from build123d import *

# Parameters (mm, degrees)
BASE_W                       = 90
BASE_H                       = 61
BASE_BLOCK_DEPTH             = 2.05
OUTER_PIN_STAND_DEPTH        = 1.4
OUTER_PIN_STAND_DEPTH_BACK   = 0.5
OUTER_PIN_R                  = 3
OUTER_PIN_STAND_2_DEPTH      = 1.4
OUTER_PIN_STAND_2_DEPTH_BACK = 0.5
OUTER_PIN_STAND_3_DEPTH      = 1.4
OUTER_PIN_STAND_3_DEPTH_BACK = 0.5
OUTER_PIN_STAND_4_DEPTH      = 1.4
OUTER_PIN_STAND_4_DEPTH_BACK = 0.5
INNER_PIN_STAND_DEPTH        = 2.6
INNER_PIN_STAND_DEPTH_BACK   = 0.5
SKETCH3_R                    = 1.25
INNER_PIN_STAND_2_DEPTH      = 2.6
INNER_PIN_STAND_2_DEPTH_BACK = 0.5
INNER_PIN_STAND_3_DEPTH      = 2.6
INNER_PIN_STAND_3_DEPTH_BACK = 0.5
INNER_PIN_STAND_4_DEPTH      = 2.6
INNER_PIN_STAND_4_DEPTH_BACK = 0.5
HOLES_DEPTH                  = 5
HOLES_DEPTH_BACK             = 5
SKETCH5_R                    = 1.75
HOLES_2_DEPTH                = 5
HOLES_2_DEPTH_BACK           = 5
SKETCH5_R_2                  = 1.775


with BuildPart() as part:
    # Base → Base Block (new body)
    with BuildSketch(Plane.XY):
        Rectangle(BASE_W, BASE_H)
    extrude(amount=-BASE_BLOCK_DEPTH)


with BuildPart() as body_2:
    # Outer Pin → Outer Pin Stand (new, two sides: drawn at the far end of the back side and taken through both)
    with BuildSketch(Plane.XY.offset(-OUTER_PIN_STAND_DEPTH_BACK)):
        with Locations((-39, 24.5)):
            Circle(OUTER_PIN_R)
    extrude(amount=OUTER_PIN_STAND_DEPTH + OUTER_PIN_STAND_DEPTH_BACK)


with BuildPart() as body_3:
    # Outer Pin → Outer Pin Stand 2 (new, two sides: drawn at the far end of the back side and taken through both)
    with BuildSketch(Plane.XY.offset(-OUTER_PIN_STAND_2_DEPTH_BACK)):
        with Locations((-39, -24.5)):
            Circle(OUTER_PIN_R)
    extrude(amount=OUTER_PIN_STAND_2_DEPTH + OUTER_PIN_STAND_2_DEPTH_BACK)


with BuildPart() as body_4:
    # Outer Pin → Outer Pin Stand 3 (new, two sides: drawn at the far end of the back side and taken through both)
    with BuildSketch(Plane.XY.offset(-OUTER_PIN_STAND_3_DEPTH_BACK)):
        with Locations((19.1, -24.5)):
            Circle(OUTER_PIN_R)
    extrude(amount=OUTER_PIN_STAND_3_DEPTH + OUTER_PIN_STAND_3_DEPTH_BACK)


with BuildPart() as body_5:
    # Outer Pin → Outer Pin Stand 4 (new, two sides: drawn at the far end of the back side and taken through both)
    with BuildSketch(Plane.XY.offset(-OUTER_PIN_STAND_4_DEPTH_BACK)):
        with Locations((19.1, 24.5)):
            Circle(OUTER_PIN_R)
    extrude(amount=OUTER_PIN_STAND_4_DEPTH + OUTER_PIN_STAND_4_DEPTH_BACK)


with BuildPart() as body_6:
    # Sketch3 → Inner Pin Stand (new, two sides: drawn at the far end of the back side and taken through both)
    with BuildSketch(Plane.XY.offset(-INNER_PIN_STAND_DEPTH_BACK)):
        with Locations((-39, 24.5)):
            Circle(SKETCH3_R)
    extrude(amount=INNER_PIN_STAND_DEPTH + INNER_PIN_STAND_DEPTH_BACK)


with BuildPart() as body_7:
    # Sketch3 → Inner Pin Stand 2 (new, two sides: drawn at the far end of the back side and taken through both)
    with BuildSketch(Plane.XY.offset(-INNER_PIN_STAND_2_DEPTH_BACK)):
        with Locations((19.1, 24.5)):
            Circle(SKETCH3_R)
    extrude(amount=INNER_PIN_STAND_2_DEPTH + INNER_PIN_STAND_2_DEPTH_BACK)


with BuildPart() as body_8:
    # Sketch3 → Inner Pin Stand 3 (new, two sides: drawn at the far end of the back side and taken through both)
    with BuildSketch(Plane.XY.offset(-INNER_PIN_STAND_3_DEPTH_BACK)):
        with Locations((19.1, -24.5)):
            Circle(SKETCH3_R)
    extrude(amount=INNER_PIN_STAND_3_DEPTH + INNER_PIN_STAND_3_DEPTH_BACK)


with BuildPart() as body_9:
    # Sketch3 → Inner Pin Stand 4 (new, two sides: drawn at the far end of the back side and taken through both)
    with BuildSketch(Plane.XY.offset(-INNER_PIN_STAND_4_DEPTH_BACK)):
        with Locations((-39, -24.5)):
            Circle(SKETCH3_R)
    extrude(amount=INNER_PIN_STAND_4_DEPTH + INNER_PIN_STAND_4_DEPTH_BACK)


with BuildPart() as body_10:
    # Sketch5 → Holes (new, two sides: drawn at the far end of the back side and taken through both)
    with BuildSketch(Plane.XY.offset(-HOLES_DEPTH_BACK)):
        with Locations((-39, -18.72)):
            Circle(SKETCH5_R)
    extrude(amount=HOLES_DEPTH + HOLES_DEPTH_BACK)


with BuildPart() as body_11:
    # Sketch5 → Holes 2 (new, two sides: drawn at the far end of the back side and taken through both)
    with BuildSketch(Plane.XY.offset(-HOLES_2_DEPTH_BACK)):
        with Locations((19.1, 18.86871886)):
            Circle(SKETCH5_R_2)
    extrude(amount=HOLES_2_DEPTH + HOLES_2_DEPTH_BACK)


with BuildPart() as part_1:
    add(part.part)

    # Combine1: union body 2, body 6, body 5, body 7, body 4, body 8, body 3, body 9
    add(body_2.part)
    add(body_6.part)
    add(body_5.part)
    add(body_7.part)
    add(body_4.part)
    add(body_8.part)
    add(body_3.part)
    add(body_9.part)

    # Combine2: cut body 11, body 10
    add(body_11.part, mode=Mode.SUBTRACT)
    add(body_10.part, mode=Mode.SUBTRACT)


solid = part_1.part
Geometry check sheet. Reference: the model listing, model coordinates, mm. A direction names the side the tool comes from. Round coordinates to 2 decimals unless told otherwise and drop trailing zeros. Order: outer loops, then holes, each group sorted by start corner. A loop starts at its lowest first (then second) coordinate and runs counter-clockwise, first axis right, second up. Notation, with made-up numbers: (-16.75, -39.75) - (19.25, -39.75) arc R23 ccw to (19.25, -31.75) - close; hole circle Ø3 at (-14, 19.25). An arc over 180 degrees is marked (long way). One line per question, with ' | ' between items. Start each with the question number.
(1) Sectioned sample at A-A on y = -18.72. Record the cut outline in (x, z).
(2) Sectioned sample at D-D on x = 5. Record the cut outline in (y, z).
(3) Sectioned sample at B-B on x = -39. Record the cut outline in (y, z).
(4) Depth check by flat-ended pin: pin 1 Ø2 at (x, y) = (-39, -18.72) entering from -Z; pin 2 Ø10 at (x, y) = (-4.5, -13.5) entering from +Z. Enter the tip coordinate at first touch or a pass-through.
(5) Sectioned sample at C-C on x = 19.1. Record the cut outline in (y, z), and give its area (3 significant figures).
(6) Release check for a two-part mould opening along X. For faces 3 (the cylindrical face through (21.87, -25.65, 0.69)), 4 (the flat face through (-1, -30.5, -1)), 5 (the flat face through (45, 0, -1)), 6 (the flat face through (19, 23, 1.4)) record: released by +X, released by -X, zero draft, split by the parting line, or undercut.
(7) Access from +Z, -Z, +X, -X, +Y, -Y to the whole of each face (thin tool, end or side, straight path). Record for faces 1 (the cylindrical face through (20.74, 18.19, -1.04)), 2 (the flat face through (-39, -26, 1.4)).
(8) Thickness scan on L1, parallel to Y at x = -39, z = -1.1; L2, parallel to X at y = -18.72, z = -0.45; L3, parallel to Y at x = 19.1, z = -0.65. Record the ranges inside material, lowest first. Write a range as [from, to].
Conclusion:
1) outline: (-45, -2.05) - (-40.75, -2.05) - (-40.75, 0) - (-45, 0) - close; (-37.25, -2.05) - (45, -2.05) - (45, 0) - (-37.25, 0) - close
2) outline: (-30.5, -2.05) - (30.5, -2.05) - (30.5, 0) - (-30.5, 0) - close
3) outline: (-30.5, -2.05) - (-20.47, -2.05) - (-20.47, 0) - (-21.5, 0) - (-21.5, 1.4) - (-23.25, 1.4) - (-23.25, 2.6) - (-25.75, 2.6) - (-25.75, 1.4) - (-27.5, 1.4) - (-27.5, 0) - (-30.5, 0) - close; (-16.97, -2.05) - (30.5, -2.05) - (30.5, 0) - (27.5, 0) - (27.5, 1.4) - (25.75, 1.4) - (25.75, 2.6) - (23.25, 2.6) - (23.25, 1.4) - (21.5, 1.4) - (21.5, 0) - (-16.97, 0) - close
4) pin 1: passes through | pin 2: stops at z = 0
5) outline: (-30.5, -2.05) - (17.09, -2.05) - (17.09, 0) - (-21.5, 0) - (-21.5, 1.4) - (-23.25, 1.4) - (-23.25, 2.6) - (-25.75, 2.6) - (-25.75, 1.4) - (-27.5, 1.4) - (-27.5, 0) - (-30.5, 0) - close; (20.64, -2.05) - (30.5, -2.05) - (30.5, 0) - (27.5, 0) - (27.5, 1.4) - (25.75, 1.4) - (25.75, 2.6) - (23.25, 2.6) - (23.25, 1.4) - (21.5, 1.4) - (21.5, 0) - (20.64, 0) - close | area: 141 mm2
6) face 3: undercut | face 4: zero draft | face 5: released by +X | face 6: undercut
7) face 1: +Z, -Z | face 2: +Z
8) L1: y = [-30.5, -20.47], [-16.97, 30.5] | L2: x = [-45, -40.75], [-37.25, 45] | L3: y = [-30.5, 17.09], [20.64, 30.5]
